```python
from build123d import *

# Parameters (mm, degrees)
SKETCH_2_R                = 2.5
CUT_EXTRUDE_1_DEPTH       = 50
CHAMFER_1_SIZE            = 2
CHAMFER_2_SIZE            = 1
CHAMFER_3_SIZE            = 1
SKETCH_3_R                = 15
CUT_EXTRUDE_2_DEPTH       = 10
HOLE_WIZARD_8_0_8_2_D     = 8
HOLE_WIZARD_8_0_8_2_DEPTH = 71
HOLE_WIZARD_8_0_8_2_TIP   = 2.403442476
M10X1_0_2_D               = 9
M10X1_0_2_DEPTH           = 20
M10X1_0_2_TIP             = 2.703872786


with BuildPart() as part:
    # 草图1 → 旋转1 (revolve)
    with BuildSketch(Plane.XY, mode=Mode.PRIVATE) as revolve_1_sk:
        with BuildLine():
            Line((0, 0), (172, 0))
            Line((172, 0), (172, 35))
            Line((172, 35), (167.5, 35))
            Line((167.5, 35), (167.5, 33))
            Line((167.5, 33), (164.8, 33))
            Line((164.8, 33), (164.8, 35))
            Line((164.8, 35), (78.358898944, 35))
            ThreePointArc((78.358898944, 35), (74, 34), (69.641101056, 35))
            Line((69.641101056, 35), (11, 35))
            Line((11, 35), (11, 30))
            Line((11, 30), (0, 30))
            Line((0, 30), (0, 0))
        make_face()
    revolve(revolve_1_sk.sketch.rotate(Axis((0, 0, 0), (1, 0, 0)), 180), axis=Axis((0, 0, 0), (1, 0, 0)))

    # 草图2 → 切除-拉伸1 (cut, symmetric)
    with BuildSketch(Plane(origin=(0, 0, 0), x_dir=(1, 0, 0), z_dir=(0, 1, 0))):
        with Locations(Location((74, 0, 0), (0, 0, 145.453943399))):
            Circle(SKETCH_2_R)
    extrude(amount=CUT_EXTRUDE_1_DEPTH, both=True, mode=Mode.SUBTRACT)

    # 倒角1
    chamfer_1_edges = [part.edges().sort_by_distance(p)[0] for p in [
        (0, 30, 0),
    ]]
    chamfer(chamfer_1_edges, length=CHAMFER_1_SIZE)

    # 倒角2
    chamfer_2_edges = [part.edges().sort_by_distance(p)[0] for p in [
        (11, 35, 0),
    ]]
    chamfer(chamfer_2_edges, length=CHAMFER_2_SIZE)

    # 倒角3
    chamfer_3_edges = [part.edges().sort_by_distance(p)[0] for p in [
        (172, 35, 0),
    ]]
    chamfer(chamfer_3_edges, length=CHAMFER_3_SIZE)

    # 草图3 → 切除-拉伸2 (cut)
    with BuildSketch(Plane.ZY):
        with Locations(Location((0, 0, 0), (0, 0, 270))):
            Circle(SKETCH_3_R)
    extrude(amount=-CUT_EXTRUDE_2_DEPTH, mode=Mode.SUBTRACT)

    # Ø8.0 (8) 直径孔2
    with Locations(Plane.ZY.offset(-10)):
        with Locations((0, 0)):
            Hole(HOLE_WIZARD_8_0_8_2_D / 2, depth=HOLE_WIZARD_8_0_8_2_DEPTH)
            with Locations((0, 0, -(HOLE_WIZARD_8_0_8_2_DEPTH + HOLE_WIZARD_8_0_8_2_TIP / 2))):  # 118° drill point
                Cone(0, HOLE_WIZARD_8_0_8_2_D / 2, HOLE_WIZARD_8_0_8_2_TIP, mode=Mode.SUBTRACT)

    # M10x1.0 螺纹孔2
    with Locations(Plane.ZY.offset(-10)):
        with Locations((0, 0)):
            Hole(M10X1_0_2_D / 2, depth=M10X1_0_2_DEPTH)
            with Locations((0, 0, -(M10X1_0_2_DEPTH + M10X1_0_2_TIP / 2))):  # 118° drill point
                Cone(0, M10X1_0_2_D / 2, M10X1_0_2_TIP, mode=Mode.SUBTRACT)


solid = part.part
```
Source: CAD feature listing. Evaluate the final solid. Frame: model axes, mm. A direction names the side the tool comes from. Round coordinates to 2 decimals unless told otherwise and drop trailing zeros. Loops run counter-clockwise (first coordinate to the right, second up) from the corner with the lowest first, then second, coordinate; pieces in that order, holes last.
1. Ray query, L1, parallel to Z at x = 52.5, y = 0; L2, parallel to Z at x = 18.5, y = 0; L3, parallel to X at y = 32, z = -6. Return the intervals inside material, ascending.
2. Section query B-B on x = 129. Output: boundary loops of the cut face in (y, z), and give its area (3 significant figures).
3. Mould query, pull axis Z, two halves, no side actions, for faces 4 (the flat face through (11, -2.4, 30.1)), 5 (the cylindrical face through (71.6, 18.9, -0.7)), 6 (the cylindrical face through (40.417, 7.587, 34.168)), 7 (the conical face through (82.986, -0.678, -0.151)). Classes: released by +Z, released by -Z, zero draft, split by the parting line, or undercut.
4. Contact query for flat-ended pins moving along their axis: pin 1 (10 mm diameter, centred on x = 103, z = -0.5, fed in from -Y); pin 2 (6 mm diameter, centred on x = 96.5, z = -10.5, fed in from +Y); pin 3 (2 mm diameter, centred on x = 53.5, z = -22.5, fed in from +Y); pin 4 (6 mm diameter, centred on x = 74, z = 0, fed in from +Y). Output: stop coordinate, or through.
5. Access query for faces 1 (the cylindrical face through (71.6, -18.5, -0.7)), 2 (the flat face through (10, -3, 4)), 3 (the flat face through (164.8, -23.5, -23.5)). Directions: +Z, -Z, +X, -X, +Y, -Y. A direction counts if a zero-diameter tool reaches every point of the face in a straight line with its end or side. Return the directions, or none.
6. Section query A-A on x = 74. Output: boundary loops of the cut face in (y, z), and give its area (3 significant figures).
Answers below:
1. L1: z = -35 to -4, 4 to 35
1. L2: z = -35 to -4.5, 4.5 to 35
1. L3: x = 11 to 172
2. outline: circle Ø70 at (0, 0)
2. area: 3,850 mm2
3. face 4: zero draft
3. face 5: undercut
3. face 6: split by the parting line
3. face 7: undercut
4. pin 1: stops at y = -35
4. pin 2: stops at y = 34.19
4. pin 3: stops at y = 27.62
4. pin 4: stops at y = 34.46
5. face 1: +Y, -Y
5. face 2: -X
5. face 3: none
6. outline: (-33.91, -2.5) arc R34 ccw to (33.91, -2.5) - (3.12, -2.5) arc R4 cw to (-3.12, -2.5) - close; (-33.91, 2.5) - (-3.12, 2.5) arc R4 cw to (3.12, 2.5) - (33.91, 2.5) arc R34 ccw to start
6. area: 3,280 mm2
